from build123d import *

# Parameters (mm, degrees)
SKETCH1_W           = 16
SKETCH1_H           = 30
SKETCH1_R           = 1.6
BOSS_EXTRUDE1_DEPTH = 3.175
SKETCH3_W           = 16
SKETCH3_H           = 22.6
BOSS_EXTRUDE2_DEPTH = 3
FILLET1_R           = 2
CUT_EXTRUDE1_DEPTH  = 52.011083355


with BuildPart() as part:
    # Sketch1 → Boss-Extrude1 (new body)
    with BuildSketch(Plane.XY):
        with Locations((0, -35)):
            Rectangle(SKETCH1_W, SKETCH1_H)
        with Locations((5, -24.85)):
            Circle(SKETCH1_R, mode=Mode.SUBTRACT)
        with Locations((-5, -24.85)):
            Circle(SKETCH1_R, mode=Mode.SUBTRACT)
    extrude(amount=BOSS_EXTRUDE1_DEPTH)

    # Sketch3 → Boss-Extrude2 (add)
    with BuildSketch(Plane(origin=(0, 0, 0), x_dir=(-1, 0, 0), z_dir=(0, 0, -1))):
        with Locations((0, -38.7)):
            Rectangle(SKETCH3_W, SKETCH3_H)
    extrude(amount=BOSS_EXTRUDE2_DEPTH)

    # Fillet1
    fillet1_edges = [part.edges().sort_by_distance(p)[0] for p in [
        (8, -50, 0.0875),
        (-8, -50, 0.0875),
    ]]
    fillet(fillet1_edges, radius=FILLET1_R)

    # Sketch4 → Cut-Extrude1 (cut, through all)
    with BuildSketch(Plane.XY.offset(3.175)):
        with BuildLine():
            Line((-8, -45), (-8, -35))
            ThreePointArc((-8, -35), (-6.244997998, -40), (-8, -45))
        make_face()
    extrude(amount=-CUT_EXTRUDE1_DEPTH, mode=Mode.SUBTRACT)


solid = part.part
CAD build for the part. Positions are in the model's coordinates, mm. A direction names the side the tool comes from. Round coordinates to 2 decimals unless told otherwise and drop trailing zeros. Loops run counter-clockwise (first coordinate to the right, second up) from the corner with the lowest first, then second, coordinate; pieces in that order, holes last. Notation, with made-up numbers: (36.25, -7) - (80.25, -7) arc R14 ccw to (80.25, 0) - close; hole circle Ø3 at (67.5, 89). An arc over 180 degrees is marked (long way). Put each result on its own line as item: value.
1. Slice it at D-D on y = -24.5. List the corners of the cut face in (x, z) (3 decimals).
Geometry check:
outline: (-8, 0) - (-6.561, 0) - (-6.561, 3.175) - (-8, 3.175) - close; (-3.439, 0) - (3.439, 0) - (3.439, 3.175) - (-3.439, 3.175) - close; (6.561, 0) - (8, 0) - (8, 3.175) - (6.561, 3.175) - close
2. 3-axis set-ups, long thin cutter, end or side, ignore diameter. For faces 5 (the flat face through (0, -27.4, -1)), 6 (the flat face through (0, -35, 3.175)): which of +Z, -Z, +X, -X, +Y, -Y reach the whole face in a straight line?
Geometry check:
face 5: -Z, +X, -X, +Y
face 6: +Z, +X, -X, +Y, -Y
3. Two-plate mould, pull along X, no slides. Class faces 1 (the flat face through (-8, -29, 1)), 2 (the cylindrical face through (-6.27, -25.82, 1.57)), 3 (the cylindrical face through (4.65, -26.41, 1.57)), 4 (the flat face through (0, -39, -3)): released by +X, released by -X, zero draft, split by the parting line, or undercut.
Geometry check:
face 1: released by -X
face 2: undercut
face 3: undercut
face 4: zero draft
4. Pin check, flat tips, straight feed: P1, Ø1.9, axis at x = -5, y = -24.85, coming from the -Z side; P2, Ø0.9, axis at x = -2.5, z = -1, coming from the +Y side. Stop position of each tip, or through.
Geometry check:
P1: through
P2: y = -27.4
5. Slice it at A-A on z = 0.5. List the corners of the cut face in (x, y) (3 decimals).
Geometry check:
outline: (-8, -48) arc R2 ccw to (-6, -50) - (6, -50) arc R2 ccw to (8, -48) - (8, -20) - (-8, -20) - (-8, -35) arc R8 cw to (-8, -45) - close; hole circle Ø3.2 at (-5, -24.85); hole circle Ø3.2 at (5, -24.85)
6. Wall check: line 1 (Y direction, x = 5, z = 0.85); line 2 (Y direction, x = -5.75, z = 2.5); line 3 (Z direction, x = -0.25, y = -26.25) (3 decimals). Give the ranges that are in metal, low to high.
Geometry check:
line 1: -50 to -26.45, -23.25 to -20
line 2: -50 to -26.26, -23.44 to -20
line 3: 0 to 3.175
7. Slice it at B-B on x = -5. List the corners of the cut face in (y, z) (3 decimals).
Geometry check:
outline: (-50, -3) - (-27.4, -3) - (-27.4, 0) - (-26.45, 0) - (-26.45, 3.175) - (-50, 3.175) - close; (-23.25, 0) - (-20, 0) - (-20, 3.175) - (-23.25, 3.175) - close
8. Slice it at C-C on z = -2. List the corners of the cut face in (x, y) (3 decimals), and give its area (3 significant figures).
Geometry check:
outline: (-8, -48) arc R2 ccw to (-6, -50) - (6, -50) arc R2 ccw to (8, -48) - (8, -27.4) - (-8, -27.4) - (-8, -35) arc R8 cw to (-8, -45) - close
area: 348 mm²
